```python
from build123d import *

# Parameters (mm, degrees)
ESTRUSIONE_ESTRUSIONE1_DEPTH = 5
SCHIZZO2_R                   = 7
TAGLIO_ESTRUSIONE1_DEPTH     = 152.6871781
RACCORDO1_R                  = 10
SCHIZZO10_R                  = 4
ESTRUSIONE_ESTRUSIONE2_DEPTH = 10
ESTRUSIONE_ESTRUSIONE2_TAPER = 14
SCHIZZO13_R                  = 4
ESTRUSIONE_ESTRUSIONE3_DEPTH = 10
ESTRUSIONE_ESTRUSIONE3_TAPER = 14


with BuildPart() as part:
    # Schizzo1 → Estrusione-Estrusione1 (new body)
    with BuildSketch(Plane.XY):
        Polygon((0, 0), (0, 78), (130, 0), align=None)
    extrude(amount=ESTRUSIONE_ESTRUSIONE1_DEPTH)

    # Schizzo2 → Taglio-Estrusione1 (cut, through all)
    with BuildSketch(Plane(origin=(0, 0, 0), x_dir=(-1, 0, 0), z_dir=(0, 0, -1))):
        with Locations((-15, 15)):
            Circle(SCHIZZO2_R)
    extrude(amount=-TAGLIO_ESTRUSIONE1_DEPTH, mode=Mode.SUBTRACT)

    # Raccordo1
    raccordo1_edges = [part.edges().sort_by_distance(p)[0] for p in [
        (0, 0, 2.5),
    ]]
    fillet(raccordo1_edges, radius=RACCORDO1_R)

    # Schizzo10 → Estrusione-Estrusione2 (add)
    with BuildSketch(Plane(origin=(0, 0, 0), x_dir=(-1, 0, 0), z_dir=(0, 0, -1))):
        with Locations((-5.463985213, 62.137606809)):
            Circle(SCHIZZO10_R)
    extrude(amount=ESTRUSIONE_ESTRUSIONE2_DEPTH, taper=ESTRUSIONE_ESTRUSIONE2_TAPER)

    # Schizzo12 → Rivoluzione1 (revolve)
    with BuildSketch(Plane.ZY.offset(-5.463985213)):
        with BuildLine():
            Line((-13, 58.137606809), (-13, 66.137606809))
            ThreePointArc((-13, 66.137606809), (-9, 62.137606809), (-13, 58.137606809))
        make_face()
    revolve(axis=Axis((5.463985213, 58.137606809, -13), (0, 1, 0)))

    # Schizzo13 → Estrusione-Estrusione3 (add)
    with BuildSketch(Plane(origin=(0, 0, 0), x_dir=(-1, 0, 0), z_dir=(0, 0, -1))):
        with Locations((-108.33809621, 6)):
            Circle(SCHIZZO13_R)
    extrude(amount=ESTRUSIONE_ESTRUSIONE3_DEPTH, taper=ESTRUSIONE_ESTRUSIONE3_TAPER)

    # Schizzo15 → Rivoluzione2 (revolve)
    with BuildSketch(Plane(origin=(31.324790173, 52.207983622, 0), x_dir=(0.8574929257125442, -0.5144957554275265, 0), z_dir=(0.5144957554275265, 0.8574929257125442, 0))):
        with BuildLine():
            Line((85.508399812, 13), (93.508399812, 13))
            ThreePointArc((93.508399812, 13), (89.508399812, 9), (85.508399812, 13))
        make_face()
    revolve(axis=Axis((104.647638101, 8.214274866, -13), (0.8574929257125445, -0.5144957554275261, 0)))


solid = part.part
```
Can you work these out from the model? Positions are in its coordinate system, mm. Coordinates: 2 decimals unless noted, no trailing zeros. Order: outer loops, then holes, each group sorted by start corner. A loop starts at its lowest first (then second) coordinate and runs counter-clockwise, first axis right, second up. Notation, with made-up numbers: (3, 3) - (29, 3) arc R24 ccw to (29, 16) - close; hole circle Ø1 at (-31, 63). An arc over 180 degrees is marked (long way). Answer in a Markdown table with one row per item.
1. For pin 1 (23.5 mm diameter, centred on x = 80.5, y = 20.5, fed in from -Z); pin 2 (10 mm diameter, centred on y = 31.5, z = -7, fed in from +X) (1 decimal); pin 3 (5 mm diameter, centred on x = 112, z = 2, fed in from +Y); pin 4 (3 mm diameter, centred on x = 111.5, z = 1, fed in from +Y), each with a flat end and sliding along its axis, tell me the tip position at first contact or that it passes through.
Reply:
| item | result |
|---|---|
| pin 1 | stops at z = 0 |
| pin 2 | passes through |
| pin 3 | stops at y = 12.3 |
| pin 4 | stops at y = 12 |
2. Suppose I cut it at B-B (x = 15). Please give me the cut outline in (y, z), and give its area (3 significant figures).
Reply:
| item | result |
|---|---|
| outline | (0, 0) - (8, 0) - (8, 5) - (0, 5) - close; (22, 0) - (69, 0) - (69, 5) - (22, 5) - close |
| area | 275 mm^2 |
3. Suppose I cut it at A-A (y = 15). Please give me the cut outline in (x, z), and give its area (3 significant figures).
Reply:
| item | result |
|---|---|
| outline | (0, 0) - (8, 0) - (8, 5) - (0, 5) - close; (22, 0) - (105, 0) - (105, 5) - (22, 5) - close |
| area | 455 mm^2 |
4. Suppose I cut it at C-C (z = -6.5). Please give me the cut outline in (x, y).
Reply:
| item | result |
|---|---|
| outline | circle Ø4.76 at (5.46, 62.14); circle Ø4.76 at (108.34, 6) |
5. If I drill on line 1 along Z through (x, y) = (65, 36.5); line 2 along Y through (x, z) = (15, 3.65); line 3 along X through (y, z) = (30, 2), over which ranges is the centre line in solid material (lowest first)?
Reply:
| item | result |
|---|---|
| line 1 | z = 0 to 5 |
| line 2 | y = 0 to 8, 22 to 69 |
| line 3 | x = 0 to 80 |
6. If we mould it in two halves opening along Z, with no side actions, what happens to faces 1 (the conical face through (105.92, 6.76, -5.87)), 2 (the flat face through (0, 44, 2)), 3 (the conical face through (5.8, 64.67, -5.79)), 4 (the flat face through (37, 22, 5))? For each: pulls with the +Z half, pulls with the -Z half, needs draft (parallel to the pull), parting line crosses it, or undercut.
Reply:
| item | result |
|---|---|
| face 1 | undercut |
| face 2 | needs draft |
| face 3 | undercut |
| face 4 | pulls with the +Z half |
7. Suppose I cut it at D-D (x = 66). Please give me the cut outline in (y, z).
Reply:
| item | result |
|---|---|
| outline | (0, 0) - (38.4, 0) - (38.4, 5) - (0, 5) - close |
